The model under review builds one solid part; all positions refer to its coordinate system, in mm. Coordinates: 2 decimals unless noted, no trailing zeros. Order: outer loops, then holes, each group sorted by start corner. A loop starts at its lowest first (then second) coordinate and runs counter-clockwise, first axis right, second up. Notation, with made-up numbers: (61.5, 68.25) -> (97.5, 68.25) arc R18 ccw to (97.5, 100.25) -> close; hole circle Ø4 at (38, 88). An arc over 180 degrees is marked (long way). Use one line per item in the form item = value.
from build123d import *

# Parameters (mm, degrees)
F0_W      = 90
F0_H      = 90
F1_DEPTH  = 1750.5
F3_DEPTH  = 4
F5_DEPTH  = 25
F7_DEPTH  = 25
F9_DEPTH  = 25
F11_DEPTH = 25
F13_DEPTH = 20


with BuildPart() as f1:
    # F0 (on Top) → F1 (new body)
    with BuildSketch(Plane.XY):
        with BuildLine():
            ThreePointArc((50, 45), (48.5355339059, 48.5355339059), (45, 50))
            Line((45, 50), (-45, 50))
            ThreePointArc((-45, 50), (-48.5355339059, 48.5355339059), (-50, 45))
            Line((-50, 45), (-50, -45))
            ThreePointArc((-50, -45), (-48.5355339059, -48.5355339059), (-45, -50))
            Line((-45, -50), (45, -50))
            ThreePointArc((45, -50), (48.5355339059, -48.5355339059), (50, -45))
            Line((50, -45), (50, 45))
        make_face()
        Rectangle(F0_W, F0_H, mode=Mode.SUBTRACT)
    extrude(amount=F1_DEPTH)

    # F2 (on face) → F3 (cut)
    with BuildSketch(Plane.XZ.offset(50)):
        with BuildLine():
            ThreePointArc((-15, 205), (-13.5355339059, 201.4644660941), (-10, 200))
            Line((-10, 200), (10, 200))
            ThreePointArc((10, 200), (13.5355339059, 201.4644660941), (15, 205))
            Line((15, 205), (15, 245))
            ThreePointArc((15, 245), (13.5355339059, 248.5355339059), (10, 250))
            Line((10, 250), (-10, 250))
            ThreePointArc((-10, 250), (-13.5355339059, 248.5355339059), (-15, 245))
            Line((-15, 245), (-15, 205))
        make_face()
    extrude(amount=-F3_DEPTH, mode=Mode.SUBTRACT)

    # F4 (on face) → F5 (cut)
    with BuildSketch(Plane(origin=(0, 50, 0), x_dir=(-1, 0, 0), z_dir=(0, 1, 0))):
        with BuildLine():
            Line((35, 1740.5), (-35, 1740.5))
            ThreePointArc((-35, 1740.5), (-38.5355339059, 1739.0355339059), (-40, 1735.5))
            Line((-40, 1735.5), (-40, 940.5))
            ThreePointArc((-40, 940.5), (-38.5355339059, 936.9644660941), (-35, 935.5))
            Line((-35, 935.5), (35, 935.5))
            ThreePointArc((35, 935.5), (38.5355339059, 936.9644660941), (40, 940.5))
            Line((40, 940.5), (40, 1735.5))
            ThreePointArc((40, 1735.5), (38.5355339059, 1739.0355339059), (35, 1740.5))
        make_face()
    extrude(amount=-F5_DEPTH, mode=Mode.SUBTRACT)

    # F6 (on face) → F7 (cut)
    with BuildSketch(Plane.XZ.offset(50)):
        with BuildLine():
            Line((7, 966), (7, 980))
            ThreePointArc((7, 980), (0, 987), (-7, 980))
            Line((-7, 980), (-7, 966))
            ThreePointArc((-7, 966), (0, 959), (7, 966))
        make_face()
        with BuildLine():
            Line((-7, 1715), (-7, 1701))
            ThreePointArc((-7, 1701), (0, 1694), (7, 1701))
            Line((7, 1701), (7, 1715))
            ThreePointArc((7, 1715), (0, 1722), (-7, 1715))
        make_face()
    extrude(amount=-F7_DEPTH, mode=Mode.SUBTRACT)

    # F8 (on face) → F9 (cut)
    with BuildSketch(Plane.YZ.offset(50)):
        with BuildLine():
            Line((45, 1000.5), (45, 1030.5))
            ThreePointArc((45, 1030.5), (43.5355339059, 1034.0355339059), (40, 1035.5))
            Line((40, 1035.5), (-10, 1035.5))
            ThreePointArc((-10, 1035.5), (-13.5355339059, 1034.0355339059), (-15, 1030.5))
            Line((-15, 1030.5), (-15, 1000.5))
            ThreePointArc((-15, 1000.5), (-13.5355339059, 996.9644660941), (-10, 995.5))
            Line((-10, 995.5), (40, 995.5))
            ThreePointArc((40, 995.5), (43.5355339059, 996.9644660941), (45, 1000.5))
        make_face()
        with BuildLine():
            Line((40, 1685.5), (-10, 1685.5))
            ThreePointArc((-10, 1685.5), (-13.5355339059, 1684.0355339059), (-15, 1680.5))
            Line((-15, 1680.5), (-15, 1650.5))
            ThreePointArc((-15, 1650.5), (-13.5355339059, 1646.9644660941), (-10, 1645.5))
            Line((-10, 1645.5), (40, 1645.5))
            ThreePointArc((40, 1645.5), (43.5355339059, 1646.9644660941), (45, 1650.5))
            Line((45, 1650.5), (45, 1680.5))
            ThreePointArc((45, 1680.5), (43.5355339059, 1684.0355339059), (40, 1685.5))
        make_face()
    extrude(amount=-F9_DEPTH, mode=Mode.SUBTRACT)

    # F10 (on face) → F11 (cut)
    with BuildSketch(Plane(origin=(-50, 0, 0), x_dir=(0, -1, 0), z_dir=(-1, 0, 0))):
        with BuildLine():
            Line((10, 1685.5), (-40, 1685.5))
            ThreePointArc((-40, 1685.5), (-43.5355339059, 1684.0355339059), (-45, 1680.5))
            Line((-45, 1680.5), (-45, 1650.5))
            ThreePointArc((-45, 1650.5), (-43.5355339059, 1646.9644660941), (-40, 1645.5))
            Line((-40, 1645.5), (10, 1645.5))
            ThreePointArc((10, 1645.5), (13.5355339059, 1646.9644660941), (15, 1650.5))
            Line((15, 1650.5), (15, 1680.5))
            ThreePointArc((15, 1680.5), (13.5355339059, 1684.0355339059), (10, 1685.5))
        make_face()
        with BuildLine():
            ThreePointArc((-40, 1035.5), (-43.5355339059, 1034.0355339059), (-45, 1030.5))
            Line((-45, 1030.5), (-45, 1000.5))
            ThreePointArc((-45, 1000.5), (-43.5355339059, 996.9644660941), (-40, 995.5))
            Line((-40, 995.5), (10, 995.5))
            ThreePointArc((10, 995.5), (13.5355339059, 996.9644660941), (15, 1000.5))
            Line((15, 1000.5), (15, 1030.5))
            ThreePointArc((15, 1030.5), (13.5355339059, 1034.0355339059), (10, 1035.5))
            Line((10, 1035.5), (-40, 1035.5))
        make_face()
    extrude(amount=-F11_DEPTH, mode=Mode.SUBTRACT)

    # F12 (on face) → F13 (join)
    with BuildSketch(Plane(origin=(0, 50, 0), x_dir=(-1, 0, 0), z_dir=(0, 1, 0))):
        with BuildLine():
            ThreePointArc((-45, 935.5), (-43.5355339059, 931.9644660941), (-40, 930.5))
            Line((-40, 930.5), (40, 930.5))
            ThreePointArc((40, 930.5), (43.5355339059, 931.9644660941), (45, 935.5))
            Line((45, 935.5), (45, 1740.3495705284))
            ThreePointArc((45, 1740.3495705284), (43.5355339059, 1743.8851044344), (40, 1745.3495705284))
            Line((40, 1745.3495705284), (-40, 1745.3495705284))
            ThreePointArc((-40, 1745.3495705284), (-43.5355339059, 1743.8851044344), (-45, 1740.3495705284))
            Line((-45, 1740.3495705284), (-45, 935.5))
        make_face()
        with BuildLine():
            Line((-40, 1735.5), (-40, 1740.3495705284))
            Line((-40, 1740.3495705284), (-36.2172369078, 1740.3495705284))
            ThreePointArc((-36.2172369078, 1740.3495705284), (-35.6132484642, 1740.4622501268), (-35, 1740.5))
            Line((-35, 1740.5), (35, 1740.5))
            ThreePointArc((35, 1740.5), (35.6132484642, 1740.4622501268), (36.2172369078, 1740.3495705284))
            Line((36.2172369078, 1740.3495705284), (40, 1740.3495705284))
            Line((40, 1740.3495705284), (40, 1735.5))
            Line((40, 1735.5), (40, 940.5))
            Line((40, 940.5), (40, 935.5))
            Line((40, 935.5), (35, 935.5))
            Line((35, 935.5), (-35, 935.5))
            Line((-35, 935.5), (-40, 935.5))
            Line((-40, 935.5), (-40, 940.5))
            Line((-40, 940.5), (-40, 1735.5))
        make_face(mode=Mode.SUBTRACT)
    extrude(amount=F13_DEPTH)


solid = f1.part
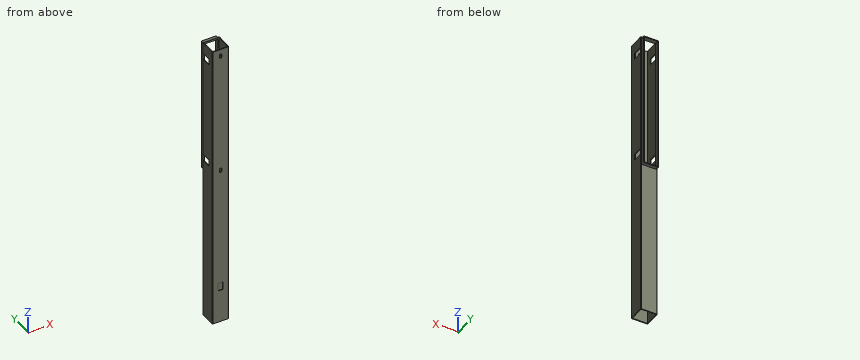
Item 1: To check wall thickness, follow L1, parallel to Y at x = 12, z = 756.5; L2, parallel to Z at x = 11.5, y = 65.5. State the ranges of each line that lie inside material, in increasing order. Write a range as from..to.
Results found:
L1 = -50..-45, 45..50
L2 = 930.5..935.5, 1740.5..1745.35
Item 2: We need section A-A (y = 16). Write out the cut boundary in (x, z).
Results found:
outline = (-50, 0) -> (-45, 0) -> (-45, 995.5) -> (-50, 995.5) -> close; (-50, 1035.5) -> (-45, 1035.5) -> (-45, 1645.5) -> (-50, 1645.5) -> close; (-50, 1685.5) -> (-45, 1685.5) -> (-45, 1750.5) -> (-50, 1750.5) -> close; (45, 0) -> (50, 0) -> (50, 995.5) -> (45, 995.5) -> close; (45, 1035.5) -> (50, 1035.5) -> (50, 1645.5) -> (45, 1645.5) -> close; (45, 1685.5) -> (50, 1685.5) -> (50, 1750.5) -> (45, 1750.5) -> close
Item 3: Clearance check with flat-ended pins moving along their axes: pin 1 (1.2 mm diameter, centred on y = -49, z = 218, fed in from -X); pin 2 (1 mm diameter, centred on y = 49.5, z = 564.5, fed in from +X); pin 3 (1.5 mm diameter, centred on x = 48, z = 1661.5, fed in from +Y). State where each tip first meets the part, or that it passes through.
Results found:
pin_1 = -48.67
pin_2 = 48
pin_3 = 49.47
Item 4: We need section B-B (z = 870). Write out the cut boundary in (x, y), plus the area to 3 significant figures.
Results found:
outline = (-50, -45) arc R5 ccw to (-45, -50) -> (45, -50) arc R5 ccw to (50, -45) -> (50, 45) arc R5 ccw to (45, 50) -> (-45, 50) arc R5 ccw to (-50, 45) -> close; hole (-45, -45) -> (45, -45) -> (45, 45) -> (-45, 45) -> close
area = 1,880 mm²
